Model file for the job. Use its own axes, mm. A direction names the side the tool comes from. Give positions to 0.01 mm unless a question says otherwise; leave off trailing zeros. Order: outer loops, then holes, each group sorted by start corner. A loop starts at its lowest first (then second) coordinate and runs counter-clockwise, first axis right, second up. Notation, with made-up numbers: (9.25, 22.5) - (60.25, 22.5) arc R23 ccw to (60.25, 48.5) - close; hole circle Ø7 at (-24, 87). An arc over 180 degrees is marked (long way). Return JSON: item names as keys, results as strings. Group by question number.
from build123d import *

# Parameters (mm, degrees)
SKETCH_W        = 213
SKETCH_H        = 333
PAD_DEPTH       = 12
SKETCH001_R     = 5.2
POCKET_DEPTH    = 5
SKETCH002_R     = 3.2
POCKET001_DEPTH = 7
FILLET_R        = 8
FILLET001_R     = 4


with BuildPart() as part:
    # Sketch → Pad (new body)
    with BuildSketch(Plane.XY):
        with Locations((106.5, 166.5)):
            Rectangle(SKETCH_W, SKETCH_H)
    extrude(amount=PAD_DEPTH)

    # Sketch001 (on Face6 of Pad) → Pocket (cut)
    with BuildSketch(Plane.XY.offset(12)):
        with Locations((16.5, 264.5)):
            Circle(SKETCH001_R)
        with Locations((16.5, 228.5)):
            Circle(SKETCH001_R)
        with Locations((16.5, 104.5)):
            Circle(SKETCH001_R)
        with Locations((16.5, 68.5)):
            Circle(SKETCH001_R)
        with Locations((196.5, 264.5)):
            Circle(SKETCH001_R)
        with Locations((196.5, 228.5)):
            Circle(SKETCH001_R)
        with Locations((196.5, 104.5)):
            Circle(SKETCH001_R)
        with Locations((196.5, 68.5)):
            Circle(SKETCH001_R)
        with Locations((106.5, 316.5)):
            Circle(SKETCH001_R)
        with Locations((106.5, 16.5)):
            Circle(SKETCH001_R)
    extrude(amount=-POCKET_DEPTH, mode=Mode.SUBTRACT)

    # Sketch002 (on Face23 of Pocket) → Pocket001 (cut)
    with BuildSketch(Plane.XY.offset(7)):
        with Locations((106.5, 316.5)):
            Circle(SKETCH002_R)
        with Locations((16.5, 264.5)):
            Circle(SKETCH002_R)
        with Locations((16.5, 228.5)):
            Circle(SKETCH002_R)
        with Locations((16.5, 104.5)):
            Circle(SKETCH002_R)
        with Locations((16.5, 68.5)):
            Circle(SKETCH002_R)
        with Locations((106.5, 16.5)):
            Circle(SKETCH002_R)
        with Locations((196.5, 68.5)):
            Circle(SKETCH002_R)
        with Locations((196.5, 104.5)):
            Circle(SKETCH002_R)
        with Locations((196.5, 228.5)):
            Circle(SKETCH002_R)
        with Locations((196.5, 264.5)):
            Circle(SKETCH002_R)
    extrude(amount=-POCKET001_DEPTH, mode=Mode.SUBTRACT)

    # Fillet
    fillet_edges = [part.edges().sort_by_distance(p)[0] for p in [
        (106.5, 0, 12),
        (213, 166.5, 12),
        (106.5, 333, 12),
        (0, 166.5, 12),
    ]]
    fillet(fillet_edges, radius=FILLET_R)

    # Fillet001
    fillet001_edges = [part.edges().sort_by_distance(p)[0] for p in [
        (0, 0, 2),
        (2.831608, 2.831608, 10.106368),
        (213, 0, 2),
        (210.168391, 2.831609, 10.106368),
        (213, 333, 2),
        (210.168392, 330.168392, 10.106368),
        (0, 333, 2),
        (2.831609, 330.168391, 10.106368),
    ]]
    fillet(fillet001_edges, radius=FILLET001_R)


solid = part.part
(1) Slice it at C-C (y = 264.5). Give the cut face in (x, z).
(2) Drill centre lines: L1, parallel to Y at x = 16.5, z = 2.5; L2, parallel to Y at x = 196.5, z = 10.5; L3, parallel to Y at x = 106.5, z = 3.5. Where is each one in solid material? Low to high.
(3) Slice it at B-B (x = 106.5). Give the cut face in (y, z), and give its area (3 significant figures).
(4) Drop flat-ended pins along their axis: pin 1 Ø5 at (y, z) = (181.5, 9) entering from -X; pin 2 Ø3 at (x, y) = (18.5, 103) entering from +Z; pin 3 Ø4 at (y, z) = (151, 10.5) entering from -X. Give the stop position or say it passes through.
(5) Pull direction Y, two halves, no side cores. Call faces 3 (the face through (107.935, 330.719, 9.594)), 4 (the face through (192.4, 261.3, 9.5)): released by +Y, released by -Y, zero draft, split by the parting line, or undercut.
(6) 3-axis set-ups, long thin cutter, end or side, ignore diameter. For faces 1 (the face through (16.083, 231.673, 3.549)), 2 (the face through (21.46, 70.06, 9.54)): which of +Z, -Z, +X, -X, +Y, -Y reach the whole face in a straight line?
(7) Slice it at D-D (x = 196.5). State how many separate pieces and enclosed holes the cut face has, and give its area (3 significant figures).
(8) Slice it at A-A (y = 316.5). Give the cut face in (x, z), and give its area (3 significant figures).
Result set:
{
 "1": {"outline": "(0, 0) - (13.3, 0) - (13.3, 7) - (11.3, 7) - (11.3, 12) - (8, 12) arc R8 ccw to (0, 4) - close; (19.7, 0) - (193.3, 0) - (193.3, 7) - (191.3, 7) - (191.3, 12) - (21.7, 12) - (21.7, 7) - (19.7, 7) - close; (199.7, 0) - (213, 0) - (213, 4) arc R8 ccw to (205, 12) - (201.7, 12) - (201.7, 7) - (199.7, 7) - close"},
 "2": {"L1": "y = 0 to 65.3, 71.7 to 101.3, 107.7 to 225.3, 231.7 to 261.3, 267.7 to 333", "L2": "y = 3.34 to 63.3, 73.7 to 99.3, 109.7 to 223.3, 233.7 to 259.3, 269.7 to 329.66", "L3": "y = 0 to 13.3, 19.7 to 313.3, 319.7 to 333"},
 "3": {"outline": "(0, 0) - (13.3, 0) - (13.3, 7) - (11.3, 7) - (11.3, 12) - (8, 12) arc R8 ccw to (0, 4) - close; (19.7, 0) - (313.3, 0) - (313.3, 7) - (311.3, 7) - (311.3, 12) - (21.7, 12) - (21.7, 7) - (19.7, 7) - close; (319.7, 0) - (333, 0) - (333, 4) arc R8 ccw to (325, 12) - (321.7, 12) - (321.7, 7) - (319.7, 7) - close", "area": "3,770 mm²"},
 "4": {"pin 1": "stops at x = 0.4", "pin 2": "stops at z = 7", "pin 3": "stops at x = 1.39"},
 "5": {"face 3": "released by +Y", "face 4": "undercut"},
 "6": {"face 1": "+Z, -Z", "face 2": "+Z"},
 "7": {"separate pieces": "5", "enclosed holes": "0", "area": "3,580 mm²"},
 "8": {"outline": "(0, 0) - (103.3, 0) - (103.3, 7) - (101.3, 7) - (101.3, 12) - (8, 12) arc R8 ccw to (0, 4) - close; (109.7, 0) - (213, 0) - (213, 4) arc R8 ccw to (205, 12) - (111.7, 12) - (111.7, 7) - (109.7, 7) - close", "area": "2,430 mm²"}
}
